```python
from build123d import *

# Parameters (mm, degrees)
SKETCH1_R           = 76.2
SKETCH1_R_2         = 38.89375
BOSS_EXTRUDE1_DEPTH = 1.5875
SKETCH3_R           = 6.35
CUT_EXTRUDE1_DEPTH  = 4.175
CIRPATTERN1_COUNT   = 5


with BuildPart() as part:
    # Sketch1 → Boss-Extrude1 (new body, symmetric)
    with BuildSketch(Plane(origin=(0, 0, 0), x_dir=(0, 0, -1), z_dir=(1, 0, 0))):
        Circle(SKETCH1_R)
        Circle(SKETCH1_R_2, mode=Mode.SUBTRACT)
    extrude(amount=BOSS_EXTRUDE1_DEPTH, both=True)

    # Sketch3 → Cut-Extrude1 (cut, through all)
    with BuildSketch(Plane(origin=(1.5875, 0, 0), x_dir=(0, 0, -1), z_dir=(1, 0, 0))):
        with Locations((0, 56.79948)):
            Circle(SKETCH3_R)
    cut_extrude1 = extrude(amount=-CUT_EXTRUDE1_DEPTH, mode=Mode.SUBTRACT)

    # CirPattern1: Cut-Extrude1 ×5 about axis
    cirpattern1_axis = Axis((0, 0, 0), (1, 0, 0))
    for i in range(1, CIRPATTERN1_COUNT):
        add(cut_extrude1.rotate(cirpattern1_axis, i * 360 / CIRPATTERN1_COUNT), mode=Mode.SUBTRACT)


solid = part.part
```
Could you check a few things on this model? Use its own coordinates, in mm. Round coordinates to 2 decimals unless told otherwise and drop trailing zeros. Write each loop counter-clockwise with the first axis right and the second up, starting at its lowest first coordinate (ties: lowest second). Pieces come first, ordered by that corner, then holes. Notation, with made-up numbers: M -32,-10 L -4,-10 A21 cw -4,29 Z; hole C 59.25,22 d8. An arc over 180 degrees is marked long. Write each question's results on one line, items separated by ' | '. Start each with the question number.
1. I need wall thicknesses on L1, parallel to Z at x = 1.3, y = 22.5; L2, parallel to Y at x = -0.75, z = 0; L3, parallel to Y at x = 0.45, z = 4. Which ranges of each line are inside material? Lowest first, please. Write a range as from..to.
2. Imagine slicing it at C-C on z = 19. List the corners of the cut face in (x, y) for me, and give its area (3 significant figures).
3. Thinking about a two-plate mould opening in Z: for faces 1 (the face through (1.588, 35, 18)), 2 (the face through (0.022, -50.559, -37.755)), 3 (the face through (0.02, 50.6, 1.38)), 4 (the face through (0.022, -46.367, 60.47)), which applies, +Z half, -Z half, draft (parallel to the pull), parting line (faces both ways), or undercut?
4. Imagine slicing it at B-B on z = 0. List the corners of the cut face in (x, y) for me.
5. I'm going to push flat-ended pins straight in: pin 1 Ø1 at (x, z) = (0.5, 31) entering from -Y; pin 2 Ø16.5 at (y, z) = (56.8, 0) entering from -X; pin 3 Ø1.5 at (x, y) = (0.5, -26) entering from +Z. Where does each tip first touch, or does it pass through?
6. Imagine slicing it at A-A on y = 0. List the corners of the cut face in (x, z) for me, and give its area (3 significant figures).
7. Imagine slicing it at D-D on x = -0.5. List the corners of the cut face in (y, z) for me, and give its area (3 significant figures).
Result sheet:
1) L1: z = -72.8..-58, -50.04..-31.72, 31.72..50.04, 58..72.8 | L2: y = -76.2..-38.89, 38.89..50.45, 63.15..76.2 | L3: y = -76.09..-38.69, 38.69..51.87, 61.73..76.09
2) outline: M -1.59,-73.79 L 1.59,-73.79 L 1.59,-33.94 L -1.59,-33.94 Z; M -1.59,33.94 L 1.59,33.94 L 1.59,73.79 L -1.59,73.79 Z | area: 253 mm^2
3) face 1: draft | face 2: undercut | face 3: undercut | face 4: parting line
4) outline: M -1.59,-76.2 L 1.59,-76.2 L 1.59,-38.89 L -1.59,-38.89 Z; M -1.59,38.89 L 1.59,38.89 L 1.59,50.45 L -1.59,50.45 Z; M -1.59,63.15 L 1.59,63.15 L 1.59,76.2 L -1.59,76.2 Z
5) pin 1: stops at y = -69.83 | pin 2: stops at x = -1.59 | pin 3: stops at z = 71.89
6) outline: M -1.59,-76.2 L 1.59,-76.2 L 1.59,-38.89 L -1.59,-38.89 Z; M -1.59,38.89 L 1.59,38.89 L 1.59,76.2 L -1.59,76.2 Z | area: 237 mm^2
7) outline: C 0,0 d152.4; hole C -45.95,-33.39 d12.7; hole C -45.95,33.39 d12.7; hole C 0,0 d77.79; hole C 17.55,-54.02 d12.7; hole C 17.55,54.02 d12.7; hole C 56.8,0 d12.7 | area: 12,900 mm^2
